Verification items for the finished model (mm, model axes). A direction names the side the tool comes from. Round coordinates to 2 decimals unless told otherwise and drop trailing zeros. Write each loop counter-clockwise with the first axis right and the second up, starting at its lowest first coordinate (ties: lowest second). Pieces come first, ordered by that corner, then holes. Notation, with made-up numbers: (-8, -5) -> (35, -5) arc R21 ccw to (35, 26) -> close; hole circle Ø8 at (88, 5.25). An arc over 180 degrees is marked (long way). Answer as a JSON object with one key per item and string values. Group by question number.
(1) Set-up check for faces 3 (the face through (8.06, 37.99, -1.96)), 4 (the face through (0, -7, 0)): record each of +Z, -Z, +X, -X, +Y, -Y from which the full face is reachable in a straight line by a thin tool's end or side.
(2) Draft check along X on faces 1 (the face through (0, 49, 0)), 2 (the face through (-8.02, 37.99, -1.95)). Enter one of: released by +X, released by -X, zero draft, split by the parting line, or undercut.
(3) Sectioned sample at C-C on y = 5. Record the cut outline in (x, z).
(4) Sectioned sample at A-A on z = 0. Record the cut outline in (x, y).
(5) Sectioned sample at B-B on x = 0. Record the cut outline in (y, z), and give its area (3 significant figures).
(6) Scan lines: L1, parallel to Y at x = -9, z = 4; L2, parallel to Z at x = -0.25, y = 6; L3, parallel to Z at x = -2.5, y = 34. Record each from-to range of solid material in increasing order. Write a range as from..to.
(7) Gauge pin test, flat ends, axial feed: pin 1 Ø1.9 at (y, z) = (-2.5, 0) entering from +X; pin 2 Ø10 at (x, y) = (0.5, 4.5) entering from -Z; pin 3 Ø6 at (x, y) = (4.5, 22) entering from +Z; pin 4 Ø1.5 at (y, z) = (32.5, -4) entering from +X. Record the tip position at first contact, or that the pin passes through.
```python
from build123d import *
from build123d.topology import SkipClean

# Parameters (mm, degrees)
SKETCH_1_R      = 2.75
EXTRUDE_1_DEPTH = 49
EXTRUDE_START   = 7
EXTRUDE_2_DEPTH = 7
EXTRUDE_START_2 = -12
SKETCH_6_R      = 11
SKETCH_6_W      = 1.25
SKETCH_6_H      = 3.5
SKETCH_6_W_2    = 3.5
SKETCH_6_H_2    = 1.25
EXTRUDE_4_DEPTH = 2


with BuildPart() as part:
    # Sketch 1 → Extrude 1 (new body)
    with BuildSketch(Plane(origin=(0, 0, 0), x_dir=(1, 0, 0), z_dir=(0, 1, 0))):
        with Locations(Location((0, 0, 0), (0, 0, 270))):
            Circle(SKETCH_1_R)
    extrude(amount=EXTRUDE_1_DEPTH)

    # Sketch 2 → Extrude 2 (add)
    with SkipClean():  # the faces are left unmerged after this step: merging them gives an invalid solid
        with BuildSketch(Plane.XZ.offset(EXTRUDE_START)):
            with BuildLine():
                Line((-1.95, 1.939071943), (-1.95, -1.939071943))
                ThreePointArc((-1.95, -1.939071943), (0, -2.75), (1.95, -1.939071943))
                Line((1.95, -1.939071943), (1.95, 1.939071943))
                ThreePointArc((1.95, 1.939071943), (0, 2.75), (-1.95, 1.939071943))
            make_face()
        extrude(amount=-EXTRUDE_2_DEPTH)

    # Sketch 6 → Extrude 4 (add)
    with SkipClean():  # the faces are left unmerged after this step: merging them gives an invalid solid
        with BuildSketch(Plane(origin=(0, 49, 0), x_dir=(1, 0, 0), z_dir=(0, 1, 0)).offset(EXTRUDE_START_2)):
            with Locations(Location((0, 0, 0), (0, 0, 270))):
                Circle(SKETCH_6_R)
            Polygon((2.495759621, 9.703700784), (3.684580266, 9.317429541), (2.603020786, 5.988731734), (1.414200141, 6.375002977), align=None, mode=Mode.SUBTRACT)
            with Locations((0, 8.25)):
                Rectangle(SKETCH_6_W, SKETCH_6_H, mode=Mode.SUBTRACT)
            Polygon((5.372216901, 8.457535726), (6.383488144, 7.722804161), (4.326239761, 4.891244681), (3.314968518, 5.625976246), align=None, mode=Mode.SUBTRACT)
            Polygon((7.722804161, 6.383488144), (8.457535726, 5.372216901), (5.625976246, 3.314968518), (4.891244681, 4.326239761), align=None, mode=Mode.SUBTRACT)
            Polygon((9.317429541, 3.684580266), (9.703700784, 2.495759621), (6.375002977, 1.414200141), (5.988731734, 2.603020786), align=None, mode=Mode.SUBTRACT)
            with Locations((8.25, 0)):
                Rectangle(SKETCH_6_W_2, SKETCH_6_H_2, mode=Mode.SUBTRACT)
            Polygon((9.703700784, -2.495759621), (9.317429541, -3.684580266), (5.988731734, -2.603020786), (6.375002977, -1.414200141), align=None, mode=Mode.SUBTRACT)
            Polygon((8.457535726, -5.372216901), (7.722804161, -6.383488144), (4.891244681, -4.326239761), (5.625976246, -3.314968518), align=None, mode=Mode.SUBTRACT)
            Polygon((6.383488144, -7.722804161), (5.372216901, -8.457535726), (3.314968518, -5.625976246), (4.326239761, -4.891244681), align=None, mode=Mode.SUBTRACT)
            Polygon((3.684580266, -9.317429541), (2.495759621, -9.703700784), (1.414200141, -6.375002977), (2.603020786, -5.988731734), align=None, mode=Mode.SUBTRACT)
            with Locations((0, -8.25)):
                Rectangle(SKETCH_6_W, SKETCH_6_H, mode=Mode.SUBTRACT)
            Polygon((-2.495759621, -9.703700784), (-3.684580266, -9.317429541), (-2.603020786, -5.988731734), (-1.414200141, -6.375002977), align=None, mode=Mode.SUBTRACT)
            Polygon((-5.372216901, -8.457535726), (-6.383488144, -7.722804161), (-4.326239761, -4.891244681), (-3.314968518, -5.625976246), align=None, mode=Mode.SUBTRACT)
            Polygon((-7.722804161, -6.383488144), (-8.457535726, -5.372216901), (-5.625976246, -3.314968518), (-4.891244681, -4.326239761), align=None, mode=Mode.SUBTRACT)
            Polygon((-9.317429541, -3.684580266), (-9.703700784, -2.495759621), (-6.375002977, -1.414200141), (-5.988731734, -2.603020786), align=None, mode=Mode.SUBTRACT)
            with Locations((-8.25, 0)):
                Rectangle(SKETCH_6_W_2, SKETCH_6_H_2, mode=Mode.SUBTRACT)
            Polygon((-9.703700784, 2.495759621), (-9.317429541, 3.684580266), (-5.988731734, 2.603020786), (-6.375002977, 1.414200141), align=None, mode=Mode.SUBTRACT)
            Polygon((-8.457535726, 5.372216901), (-7.722804161, 6.383488144), (-4.891244681, 4.326239761), (-5.625976246, 3.314968518), align=None, mode=Mode.SUBTRACT)
            Polygon((-6.383488144, 7.722804161), (-5.372216901, 8.457535726), (-3.314968518, 5.625976246), (-4.326239761, 4.891244681), align=None, mode=Mode.SUBTRACT)
            Polygon((-3.684580266, 9.317429541), (-2.495759621, 9.703700784), (-1.414200141, 6.375002977), (-2.603020786, 5.988731734), align=None, mode=Mode.SUBTRACT)
        extrude(amount=EXTRUDE_4_DEPTH)


solid = part.part
```
Computed values:
{
 "1": {"face 3": "+Y, -Y", "face 4": "+Z, -Z, +X, -X, -Y"},
 "2": {"face 1": "zero draft", "face 2": "undercut"},
 "3": {"outline": "circle Ø5.5 at (0, 0)"},
 "4": {"outline": "(-11, 37) -> (-10, 37) -> (-10, 39) -> (-11, 39) -> close; (-6.5, 37) -> (-2.75, 37) -> (-2.75, 0) -> (-1.95, 0) -> (-1.95, -7) -> (1.95, -7) -> (1.95, 0) -> (2.75, 0) -> (2.75, 37) -> (6.5, 37) -> (6.5, 39) -> (2.75, 39) -> (2.75, 49) -> (-2.75, 49) -> (-2.75, 39) -> (-6.5, 39) -> close; (10, 37) -> (11, 37) -> (11, 39) -> (10, 39) -> close"},
 "5": {"outline": "(-7, -2.75) -> (37, -2.75) -> (37, -6.5) -> (39, -6.5) -> (39, -2.75) -> (49, -2.75) -> (49, 2.75) -> (39, 2.75) -> (39, 6.5) -> (37, 6.5) -> (37, 2.75) -> (-7, 2.75) -> close; (37, -11) -> (39, -11) -> (39, -10) -> (37, -10) -> close; (37, 10) -> (39, 10) -> (39, 11) -> (37, 11) -> close", "area": "327 mm2"},
 "6": {"L1": "37..39", "L2": "-2.74..2.74", "L3": "-1.15..1.15"},
 "7": {"pin 1": "x = 1.95", "pin 2": "z = -2.75", "pin 3": "z = 2.3", "pin 4": "through"}
}
